```python
from build123d import *

# Parameters (mm, degrees)
SKETCH4_W               = 0.254
SKETCH4_H               = 0.254
SKETCH4_W_2             = 1.778
CUT_EXTRUDE1_DEPTH      = 0.508
CUT_EXTRUDE2_DEPTH      = 0.508
CUT_EXTRUDE3_DEPTH      = 0.508
SKETCH8_W               = 1.524
SKETCH8_H               = 1.016
SKETCH8_W_2             = 2.54
SKETCH8_H_2             = 0.508
CUT_EXTRUDE4_DEPTH      = 1.0000001
CUT_EXTRUDE4_DEPTH_BACK = 0.508


with BuildPart() as part:
    # Sketch1 → Loft1 section 0
    with BuildSketch(Plane(origin=(0, 0, 0), x_dir=(1, 0, 0), z_dir=(0, 1, 0)), mode=Mode.PRIVATE) as loft1_s0:
        Polygon((0, 7.332348419), (-6.35, -3.666174209), (6.35, -3.666174209), align=None)
    loft([Vertex(0, 10.414, 0), loft1_s0.sketch])

    # Sketch4 → Cut-Extrude1 (cut)
    with BuildSketch(Plane(origin=(0, 1.148332745, 3.26191188), x_dir=(1, 0, 0), z_dir=(0, 0.332066518, 0.943255972))):
        Polygon((1.016, 2.846586297), (1.016, 2.592586297), (1.016, 2.338586297), (1.016, 1.322586297), (-1.016, 1.322586297), (-1.016, 1.068586297), (1.27, 1.068586297), (1.27, 2.592586297), (1.27, 4.116586297), (-1.016, 4.116586297), (-1.016, 3.862586297), (1.016, 3.862586297), align=None)
        Polygon((0.762, 3.608586297), (0.762, 2.846586297), (1.016, 2.846586297), (1.016, 3.862586297), (-1.016, 3.862586297), (-1.016, 3.608586297), align=None)
        with Locations((0.889, 2.719586297)):
            Rectangle(SKETCH4_W, SKETCH4_H)
        with Locations((0.889, 2.465586297)):
            Rectangle(SKETCH4_W, SKETCH4_H)
        with Locations((-0.127, 2.719586297)):
            Rectangle(SKETCH4_W_2, SKETCH4_H)
        with Locations((-0.127, 2.465586297)):
            Rectangle(SKETCH4_W_2, SKETCH4_H)
        Polygon((1.016, 2.338586297), (0.762, 2.338586297), (0.762, 1.576586297), (-1.016, 1.576586297), (-1.016, 1.322586297), (1.016, 1.322586297), align=None)
    extrude(amount=-CUT_EXTRUDE1_DEPTH, mode=Mode.SUBTRACT)

    # Sketch6 → Cut-Extrude2 (cut)
    with BuildSketch(Plane(origin=(2.824898553, 1.148332745, -1.63095594), x_dir=(-0.436908848, -0.177605223, -0.88179762), z_dir=(0.816883634, 0.332066518, -0.471627986))):
        Polygon((-1.523480632, 3.899478619), (-2.022394323, 3.803827539), (-1.68761554, 2.057629621), (0.308039223, 2.440233945), (0.642818006, 0.694036027), (1.141731697, 0.789687108), (0.47217413, 4.282082943), (-0.02673956, 4.186431862), (0.212388142, 2.939147635), (-1.28435293, 2.652194393), align=None)
    extrude(amount=-CUT_EXTRUDE2_DEPTH, mode=Mode.SUBTRACT)

    # Sketch7 → Cut-Extrude3 (cut)
    with BuildSketch(Plane(origin=(-2.824898553, 1.148332745, -1.63095594), x_dir=(-0.436908848, 0.177605223, 0.88179762), z_dir=(-0.816883634, 0.332066518, -0.471627986))):
        Polygon((-0.844449311, 0.991318413), (1.400662297, 0.560888549), (1.73544108, 2.307086467), (-0.260213682, 2.68969079), (-0.116737061, 3.438061326), (1.629460856, 3.103282543), (1.725111937, 3.602196234), (-0.519999671, 4.032626098), (-0.854778454, 2.28642818), (1.140876309, 1.903823857), (0.997399687, 1.155453321), (-0.74879823, 1.490232104), align=None)
    extrude(amount=-CUT_EXTRUDE3_DEPTH, mode=Mode.SUBTRACT)

    # Sketch8 → Cut-Extrude4 (cut, two sides)
    with BuildSketch(Plane.XZ) as cut_extrude4_sk:
        Polygon((-1.016, -1.27), (-1.016, -1.778), (1.27, -1.778), (1.27, 1.778), (-1.27, 1.778), (-1.27, -0.254), (0.762, -0.254), (0.762, -1.27), align=None)
        with Locations((0, 0.762)):
            Rectangle(SKETCH8_W, SKETCH8_H, mode=Mode.SUBTRACT)
        with Locations((0, 2.794)):
            Rectangle(SKETCH8_W_2, SKETCH8_H_2)
    extrude(amount=CUT_EXTRUDE4_DEPTH, mode=Mode.SUBTRACT)
    extrude(cut_extrude4_sk.sketch, amount=-CUT_EXTRUDE4_DEPTH_BACK, mode=Mode.SUBTRACT)


solid = part.part
```
Geometry check sheet. Reference: the model listing, model coordinates, mm. A direction names the side the tool comes from. Give positions to 0.01 mm unless a question says otherwise; leave off trailing zeros. Order: outer loops, then holes, each group sorted by start corner. A loop starts at its lowest first (then second) coordinate and runs counter-clockwise, first axis right, second up. Notation, with made-up numbers: (18, 35.5) - (39, 35.5) arc R8 ccw to (39, 46.5) - close; hole circle Ø1 at (-31.75, -0.75). An arc over 180 degrees is marked (long way). Write item = value, one per line. Start each with the question number.
1) Section check C-C (y = 8.5). Enter the section's corners in (x, z), then the cut area to 3 significant figures.
2) Section check A-A (z = 1). Enter the section's corners in (x, y).
3) Draft check along X on faces 1 (the flat face through (-2.18, 2.31, -1.39)), 2 (the flat face through (1.82, 2.44, -1.93)), 3 (the flat face through (2.007, 3.977, -1.056)), 4 (the flat face through (2, 0, 1)). Enter one of: released by +X, released by -X, zero draft, split by the parting line, or undercut.
4) Access from +Z, -Z, +X, -X, +Y, -Y to the whole of each face (thin tool, end or side, straight path). Record for faces 5 (the flat face through (-1.918, 3.977, -1.21)), 6 (the flat face through (-1.71, 4.23, -0.86)).
5) Scan lines: L1, parallel to Y at x = 0.5, z = -4.25; L2, parallel to Y at x = 2, z = -0.75; L3, parallel to Z at x = 1, y = 1.5. Record each from-to range of solid material in increasing order.
6) Gauge pin test, flat ends, axial feed: pin 1 Ø0.6 at (x, y) = (-0.5, 0.5) entering from -Z; pin 2 Ø5 at (y, z) = (6.5, -4) entering from -X; pin 3 Ø1.3 at (x, z) = (-0.5, 0) entering from -Y; pin 4 Ø1.5 at (x, y) = (0.5, 6.5) entering from -Z. Record the tip position at first contact, or that the pin passes through.
7) Section check B-B (x = -3). Enter the section's corners in (y, z).
8) Section check D-D (z = -1). Enter the section's corners in (x, y).
Geometry check:
q1.outline = (-1.17, 0.67) - (0, -1.35) - (1.17, 0.67) - close
q1.area = 2.36 mm2
q2.outline = (-4.81, 0) - (-1.27, 0) - (-1.27, 0.51) - (-0.76, 0.51) - (-0.76, 0) - (0.76, 0) - (0.76, 0.51) - (1.27, 0.51) - (1.27, 0) - (4.81, 0) - (1.73, 7.57) - (-1.73, 7.57) - close
q3.face_1 = released by -X
q3.face_2 = undercut
q3.face_3 = released by +X
q3.face_4 = zero draft
q4.face_5 = -Z, -X, +Y
q4.face_6 = none
q5.L1 = 0 to 3.15
q5.L2 = 0 to 3.22, 3.76 to 4.43
q5.L3 = -4.54 to 3.14
q6.pin_1 = -6.68
q6.pin_2 = -1.05
q6.pin_3 = 0
q6.pin_4 = -3.15
q7.outline = (0, -2.14) - (1.92, -0.79) - (1.82, -0.27) - (2.66, -0.27) - (5.49, 1.73) - (0, 3.67) - close
q8.outline = (-3.66, 0) - (0.76, 0) - (0.76, 0.51) - (1.27, 0.51) - (1.27, 0) - (3.66, 0) - (2.29, 3.35) - (1.74, 3.19) - (1.54, 3.66) - (2.1, 3.83) - (0, 8.99) - (-1.71, 4.79) - (-1.15, 4.62) - (-1.35, 4.14) - (-1.9, 4.31) - (-2.2, 3.59) - (-1.64, 3.43) - (-1.84, 2.95) - (-2.39, 3.11) - (-2.68, 2.4) - (-2.13, 2.23) - (-2.32, 1.75) - (-2.88, 1.92) - close
